```python
from build123d import *

# Parameters (mm, degrees)
ESBO_O2_R                = 25
ESBO_O3_R                = 6
RESSALTO_EXTRUS_O1_DEPTH = 35
ESBO_O4_R                = 6
CORTE_EXTRUS_O1_DEPTH    = 20


with BuildPart() as part:
    # Varredura1: sweep along a path in Esboço1
    with BuildLine(Plane.XY) as varredura1_path:
        Line((13.022726178, 77.820743024), (0, 40))
        Line((0, 40), (0, 0))
    # Esboço2 → Varredura1 (sweep)
    with BuildSketch(Plane(origin=(0, 0, 0), x_dir=(1, 0, 0), z_dir=(0, 1, 0))):
        Circle(ESBO_O2_R)
    sweep(path=varredura1_path.line, transition=Transition.RIGHT)

    # Esboço3 → Ressalto-extrusão1 (add)
    with BuildSketch(Plane(origin=(25.335955685, 73.580958096, 0), x_dir=(0.945518576, -0.325568154, 0), z_dir=(0.325568154, 0.945518576, 0))):
        with Locations((-13.022726178, 0)):
            Circle(ESBO_O3_R)
    extrude(amount=RESSALTO_EXTRUS_O1_DEPTH)

    # Esboço4 → Corte-extrusão1 (cut)
    with BuildSketch(Plane.XZ):
        Circle(ESBO_O4_R)
    extrude(amount=-CORTE_EXTRUS_O1_DEPTH, mode=Mode.SUBTRACT)


solid = part.part
```
Can you work these out from the model? Positions are in its coordinate system, mm. A direction names the side the tool comes from. Coordinates: 2 decimals unless noted, no trailing zeros. Loops run counter-clockwise (first coordinate to the right, second up) from the corner with the lowest first, then second, coordinate; pieces in that order, holes last. Notation, with made-up numbers: (-35, 5) -> (-26, 5) arc R30 cw to (-26, 41) -> close; hole circle Ø9 at (8.25, 17). An arc over 180 degrees is marked (long way). Answer as a JSON object with one key per item and string values.
1) Imagine slicing it at B-B (y = 22.5). Please give me the cut outline in (x, z), then the cut area to 3 significant figures.
Results:
{"outline": "circle Ø50 at (0, 0)", "area": "1,960 mm^2"}
2) For P1, Ø8, axis at x = -11, y = 21, coming from the -Z side; P2, Ø2, axis at x = 16.5, z = 17.5, coming from the +Y side; P3, Ø6, axis at y = 59.5, z = 9.5, coming from the -X side, each with a flat end and sliding along its axis, tell me the tip position at first contact or that it passes through.
Results:
{"P1": "stops at z = -24", "P2": "stops at y = 76.97", "P3": "stops at x = -19.28"}
3) Thinking about a two-plate mould opening in X: for faces 3 (the face through (-24.976, 21.782, 1.099)), 4 (the face through (-5, 0, 5)), 5 (the face through (-6, 10, 0)), which applies, pulls with the +X half, pulls with the -X half, needs draft (parallel to the pull), parting line crosses it, or undercut?
Results:
{"face 3": "parting line crosses it", "face 4": "needs draft", "face 5": "undercut"}
4) For faces 1 (the face through (-17.885, 64.771, 1.099)), 2 (the face through (0, 20, 0)), which set-ups out of +Z, -Z, +X, -X, +Y, -Y let a thin tool reach every point of the face, with its end or its side?
Results:
{"face 1": "none", "face 2": "-Y"}
5) Imagine slicing it at C-C (z = 0). Please give me the cut outline in (x, y).
Results:
{"outline": "(-25, 0) -> (-6, 0) -> (-6, 20) -> (6, 20) -> (6, 0) -> (25, 0) -> (25, 35.82) -> (36.66, 69.68) -> (18.7, 75.87) -> (30.09, 108.96) -> (18.74, 112.87) -> (7.35, 79.77) -> (-10.62, 85.96) -> (-25, 44.18) -> close"}
6) Imagine slicing it at D-D (z = 19.5). Please give me the cut outline in (x, y).
Results:
{"outline": "(-15.64, 0) -> (15.64, 0) -> (15.64, 37.38) -> (27.81, 72.73) -> (-1.77, 82.91) -> (-15.64, 42.62) -> close"}
7) Imagine slicing it at A-A (y = 10.5). Please give me the cut outline in (x, z), then the cut area to 3 significant figures.
Results:
{"outline": "circle Ø50 at (0, 0); hole circle Ø12 at (0, 0)", "area": "1,850 mm^2"}
8) If I drill on line 1 (Z direction, x = 0, y = 7.5); line 2 (X direction, y = 62.5, z = -18.5); line 3 (X direction, y = 53.5, z = 13.5), over which ranges is the centre line in solid material (lowest first)?
Results:
{"line 1": "z = -25 to -6, 6 to 25", "line 2": "x = -10.04 to 25.53", "line 3": "x = -17.61 to 26.9"}
